from build123d import *

# Parameters (mm, degrees)
SKETCH1_W           = 38.1
SKETCH1_H           = 38.1
SKETCH1_R           = 1.5875
BOSS_EXTRUDE2_DEPTH = 15.24
SKETCH3_R           = 3.175
BOSS_EXTRUDE3_DEPTH = 19.05
FILLET2_R           = 2.54
CHAMFER1_SIZE       = 1.27
SKETCH4_R           = 2.413
CUT_EXTRUDE2_DEPTH  = 7.62
SKETCH5_R           = 2.413
CUT_EXTRUDE3_DEPTH  = 7.62


with BuildPart() as part:
    # Sketch1 → Boss-Extrude2 (new body)
    with BuildSketch(Plane.XY):
        Rectangle(SKETCH1_W, SKETCH1_H)
        Circle(SKETCH1_R, mode=Mode.SUBTRACT)
    extrude(amount=BOSS_EXTRUDE2_DEPTH)

    # Sketch3 → Boss-Extrude3 (add)
    with BuildSketch(Plane.XY.offset(15.24)):
        Circle(SKETCH3_R)
    extrude(amount=BOSS_EXTRUDE3_DEPTH)

    # Fillet2
    fillet2_edges = [part.edges().sort_by_distance(p)[0] for p in [
        (-19.05, 19.05, 7.62),
        (19.05, 19.05, 7.62),
        (19.05, -19.05, 7.62),
        (-19.05, -19.05, 7.62),
    ]]
    fillet(fillet2_edges, radius=FILLET2_R)

    # Chamfer1
    chamfer1_edges = [part.edges().sort_by_distance(p)[0] for p in [
        (-3.175, 0, 34.29),
    ]]
    chamfer(chamfer1_edges, length=CHAMFER1_SIZE)

    # Sketch4 → Cut-Extrude2 (cut)
    with BuildSketch(Plane.XZ.offset(19.05)):
        with Locations((-9.525, 7.62)):
            Circle(SKETCH4_R)
        with Locations((9.525, 7.62)):
            Circle(SKETCH4_R)
    extrude(amount=-CUT_EXTRUDE2_DEPTH, mode=Mode.SUBTRACT)

    # Sketch5 → Cut-Extrude3 (cut)
    with BuildSketch(Plane(origin=(0, 19.05, 0), x_dir=(1, 0, 0), z_dir=(0, 1, 0))):
        with Locations((9.525, -7.62)):
            Circle(SKETCH5_R)
        with Locations((-9.525, -7.62)):
            Circle(SKETCH5_R)
    extrude(amount=-CUT_EXTRUDE3_DEPTH, mode=Mode.SUBTRACT)


solid = part.part
The model under review builds one solid part; all positions refer to its coordinate system, in mm. A direction names the side the tool comes from. Give positions to 0.01 mm unless a question says otherwise; leave off trailing zeros. Write each loop counter-clockwise with the first axis right and the second up, starting at its lowest first coordinate (ties: lowest second). Pieces come first, ordered by that corner, then holes.
1. Tool access review of faces 4 (the cylindrical face through (-11.303, 15.293, 5.989)), 5 (the cylindrical face through (-0.69, -3.1, 24.01)), 6 (the flat face through (19.05, 0, 8)), 7 (the cylindrical face through (-0.34, -1.55, 7.51)), 8 (the flat face through (-10, -11.43, 8)): name each direction out of +Z, -Z, +X, -X, +Y, -Y from which nothing blocks a thin tool from reaching the whole face with its end or side.
2. Wall thickness on L1, parallel to X at y = 16, z = 7.62; L2, parallel to Y at x = 0, z = 11; L3, parallel to Z at x = 6.5, y = 16: over which ranges is each line inside the solid? List them lowest first.
3. Add section A-A, the plane y = 14. Write out the cut boundary in (x, z) (3 decimals).
4. For P1, Ø2, axis at x = 4, y = 2, coming from the +Z side; P2, Ø4, axis at x = -9.525, z = 7.62, coming from the -Y side; P3, Ø5.5, axis at x = -10.5, z = 7, coming from the -Y side; P4, Ø4.5, axis at x = -9.525, z = 7.62, coming from the +Y side, all flat-tipped, find the tip position at first contact; note any pin that passes through.
5. Draft analysis for pull direction X (two halves, no side actions). For faces 1 (the cylindrical face through (-18.326, -18.286, 7.727)), 2 (the cylindrical face through (18.286, -18.326, 7.727)), 3 (the cylindrical face through (10.822, 15.293, 5.585)), state which applies: +X half, -X half, draft (parallel to the pull), parting line (faces both ways), or undercut.
Worked answers:
1. face 4: +Y
1. face 5: +Z
1. face 6: +Z, -Z, +X, +Y, -Y
1. face 7: -Z
1. face 8: -Y
2. L1: x = -19.05 to -11.94, -7.11 to 7.11, 11.94 to 19.05
2. L2: y = -19.05 to -1.59, 1.59 to 19.05
2. L3: z = 0 to 15.24
3. outline: (-19.05, 0) - (19.05, 0) - (19.05, 15.24) - (-19.05, 15.24) - close; hole circle Ø4.826 at (-9.525, 7.62); hole circle Ø4.826 at (9.525, 7.62)
4. P1: stops at z = 15.24
4. P2: stops at y = -11.43
4. P3: stops at y = -19.05
4. P4: stops at y = 11.43
5. face 1: -X half
5. face 2: +X half
5. face 3: undercut
